```python
from build123d import *

# Parameters (mm, degrees)
BOSS_EXTRUDE1_DEPTH = 2.5


with BuildPart() as part:
    # Sketch2 → Boss-Extrude1 (new, symmetric)
    with BuildSketch(Plane.XY):
        Polygon((-366.252975542, -70.079481859), (-376.502975542, -70.079481859), (-376.502975542, -75.579481859), (-366.252975542, -75.579481859), (-366.252975542, -133.729086599), (-361.252975542, -133.729086599), (-361.252975542, -144.729086599), (-356.252975542, -144.729086599), (-341.252975542, -148.729086599), (-341.252975542, -153.729086599), (-386.252975542, -153.729086599), (-386.252975542, 5.770882486), (-341.252975542, 5.770882486), (-341.252975542, 0.770882486), (-356.252975542, -3.229117514), (-361.252975542, -3.229117514), (-361.252975542, -14.229117514), (-366.252975542, -14.229117514), align=None)
    extrude(amount=BOSS_EXTRUDE1_DEPTH, both=True)


solid = part.part
```
For this review, take the finished solid that the model builds, in its own axes (mm). A direction names the side the tool comes from. Coordinates: 2 decimals unless noted, no trailing zeros. Order: outer loops, then holes, each group sorted by start corner. A loop starts at its lowest first (then second) coordinate and runs counter-clockwise, first axis right, second up. Notation, with made-up numbers: (-22.5, 34.5) -> (-3.5, 34.5) arc R31 ccw to (-3.5, 63.5) -> close; hole circle Ø8 at (20, -12.75). An arc over 180 degrees is marked (long way). Answer as CSV lines item,"result".
Q1. For faces 5 (the face through (-341.253, -151, 0)), 6 (the face through (-366.253, -42, 0)), list the 3-axis set-ups (+Z, -Z, +X, -X, +Y, -Y) from which the entire face can be reached by the end or side of a thin tool; tool diameter is ignored.
Model answer:
face 5,"+Z, -Z, +X, +Y, -Y"
face 6,"+Z, -Z, +X"
Q2. We need section D-D (y = -141.5). State the section outline as (x, z) points, plus the area to 3 significant figures.
Model answer:
outline,"(-386.25, -2.5) -> (-361.25, -2.5) -> (-361.25, 2.5) -> (-386.25, 2.5) -> close"
area,"125 mm2"
Q3. We need section C-C (x = -363.5). State the section outline as (y, z) points.
Model answer:
outline,"(-153.73, -2.5) -> (-133.73, -2.5) -> (-133.73, 2.5) -> (-153.73, 2.5) -> close; (-14.23, -2.5) -> (5.77, -2.5) -> (5.77, 2.5) -> (-14.23, 2.5) -> close"
Q4. We need section B-B (z = -1.1). State the section outline as (x, y) points, plus the area to 3 significant figures.
Model answer:
outline,"(-386.25, -153.73) -> (-341.25, -153.73) -> (-341.25, -148.73) -> (-356.25, -144.73) -> (-361.25, -144.73) -> (-361.25, -133.73) -> (-366.25, -133.73) -> (-366.25, -75.58) -> (-376.5, -75.58) -> (-376.5, -70.08) -> (-366.25, -70.08) -> (-366.25, -14.23) -> (-361.25, -14.23) -> (-361.25, -3.23) -> (-356.25, -3.23) -> (-341.25, 0.77) -> (-341.25, 5.77) -> (-386.25, 5.77) -> close"
area,"3,630 mm2"
Q5. Wall thickness on line 1 along Y through (x, z) = (-374.5, 0.8); line 2 along Y through (x, z) = (-363, -2.25); line 3 along X through (y, z) = (-137, -0.5): over which ranges is each line inside the solid? List them lowest first. Write a range as [from, to].
Model answer:
line 1,"y = [-153.73, -75.58], [-70.08, 5.77]"
line 2,"y = [-153.73, -133.73], [-14.23, 5.77]"
line 3,"x = [-386.25, -361.25]"
Q6. Draft analysis for pull direction Y (two halves, no side actions). For faces 1 (the face through (-378, -73, -2.5)), 2 (the face through (-363, -153.729, 0)), 3 (the face through (-364, 5.771, 0)), 4 (the face through (-361.253, -9, 0)), state which applies: released by +Y, released by -Y, zero draft, split by the parting line, or undercut.
Model answer:
face 1,"zero draft"
face 2,"released by -Y"
face 3,"released by +Y"
face 4,"undercut"
Q7. Clearance check with flat-ended pins moving along their axes: pin 1 Ø2 at (y, z) = (-75.5, -0.5) entering from +X; pin 2 Ø1.5 at (y, z) = (-11, -0.5) entering from +X; pin 3 Ø1.5 at (y, z) = (-73, -1) entering from +X. State where each tip first meets the part, or that it passes through.
Model answer:
pin 1,"stops at x = -366.25"
pin 2,"stops at x = -361.25"
pin 3,"stops at x = -376.5"
Q8. We need section A-A (x = -372). State the section outline as (y, z) points.
Model answer:
outline,"(-153.73, -2.5) -> (-75.58, -2.5) -> (-75.58, 2.5) -> (-153.73, 2.5) -> close; (-70.08, -2.5) -> (5.77, -2.5) -> (5.77, 2.5) -> (-70.08, 2.5) -> close"
